```python
from build123d import *

# Parameters (mm, degrees)
F1_DEPTH = 76.2
F3_DEPTH = 50.8
F5_DEPTH = 25.4


with BuildPart() as f1:
    # F0 (on Front) → F1 (new body)
    with BuildSketch(Plane.XZ):
        Polygon((0, 50.8), (0, 0), (152.4, 0), (152.4, 25.4), (25.4, 25.4), (25.4, 50.8), align=None)
    extrude(amount=F1_DEPTH)

    # F2 (on face) → F3 (join)
    with BuildSketch(Plane.XZ.offset(76.2)):
        Polygon((152.4, 25.4), (25.4, 50.8), (25.4, 25.4), align=None)
    extrude(amount=-F3_DEPTH)

    # F4 (on face) → F5 (cut)
    with BuildSketch(Plane.XZ.offset(76.2)):
        Polygon((152.4, 25.4), (25.4, 50.8), (25.4, 28.610824), align=None)
    extrude(amount=-F5_DEPTH, mode=Mode.SUBTRACT)


solid = f1.part
```
Input: part model. Units: mm. Frame: model coordinates. A direction names the side the tool comes from. Give positions to 0.01 mm unless a question says otherwise; leave off trailing zeros. Order: outer loops, then holes, each group sorted by start corner. A loop starts at its lowest first (then second) coordinate and runs counter-clockwise, first axis right, second up.
1. Section C-C on y = -15.5. Return the cut outline in (x, z), and give its area (3 significant figures).
Derived:
outline: (0, 0) - (152.4, 0) - (152.4, 25.4) - (25.4, 25.4) - (25.4, 50.8) - (0, 50.8) - close
area: 4,520 mm2
2. Section A-A on z = 44. Return the cut outline in (x, y), and give its area (3 significant figures).
Derived:
outline: (0, -76.2) - (25.4, -76.2) - (25.4, -50.8) - (59.4, -50.8) - (59.4, -25.4) - (25.4, -25.4) - (25.4, 0) - (0, 0) - close
area: 2,800 mm2
3. Reachability of faces 1 (the flat face through (25.4, -13, 38)), 2 (the flat face through (25.4, -64, 40)), 3 (the flat face through (0, -38, 26)) from +Z, -Z, +X, -X, +Y, -Y: full face, straight path, thin tool, end or side. Return the list, or none.
Derived:
face 1: +Z, +X, +Y
face 2: +Z, +X, -Y
face 3: +Z, -Z, -X, +Y, -Y
4. Section B-B on x = 113.5. Return the cut outline in (y, z).
Derived:
outline: (-76.2, 0) - (0, 0) - (0, 25.4) - (-25.4, 25.4) - (-25.4, 33.18) - (-50.8, 33.18) - (-50.8, 26.38) - (-76.2, 26.38) - close
5. Pin query (flat end, axial travel): pin 1 (11 mm diameter, centred on y = -64, z = 38, fed in from +X); pin 2 (12 mm diameter, centred on x = 88, y = -32, fed in from +Z); pin 3 (20.5 mm diameter, centred on x = 88, z = 40.5, fed in from +Y). Return the tip coordinate at first contact, or that it passes through.
Derived:
pin 1: stops at x = 25.4
pin 2: stops at z = 39.48
pin 3: stops at y = -25.4
6. Material intervals for L1, parallel to Y at x = 38, z = 35.5; L2, parallel to Z at x = 52, y = -20.5, sorted ascending.
Derived:
L1: y = -50.8 to -25.4
L2: z = 0 to 25.4
7. Section D-D on y = -69. Return the cut outline in (x, z).
Derived:
outline: (0, 0) - (152.4, 0) - (152.4, 25.4) - (25.4, 28.61) - (25.4, 50.8) - (0, 50.8) - close
